from build123d import *

# Parameters (mm, degrees)
SKETCH2_R           = 42.5
BOSS_EXTRUDE2_DEPTH = 75
SKETCH3_R           = 27.5
BOSS_EXTRUDE3_DEPTH = 40
SKETCH4_W           = 10.5
SKETCH4_H           = 8.79879656
CUT_EXTRUDE1_DEPTH  = 50


with BuildPart() as part:
    # Sketch2 → Boss-Extrude2 (new, symmetric)
    with BuildSketch(Plane.XY):
        Circle(SKETCH2_R)
    extrude(amount=BOSS_EXTRUDE2_DEPTH, both=True)

    # Sketch3 → Boss-Extrude3 (add)
    with BuildSketch(Plane.XY.offset(75)):
        Circle(SKETCH3_R)
    boss_extrude3 = extrude(amount=BOSS_EXTRUDE3_DEPTH)

    # Sketch4 → Cut-Extrude1 (cut, symmetric)
    with BuildSketch(Plane(origin=(0, 0, 0), x_dir=(0, 0, -1), z_dir=(1, 0, 0))):
        with Locations((-96.25, 24.39939828)):
            Rectangle(SKETCH4_W, SKETCH4_H)
    cut_extrude1 = extrude(amount=CUT_EXTRUDE1_DEPTH, both=True, mode=Mode.SUBTRACT)

    # Mirror3: Boss-Extrude3, Cut-Extrude1 across plane
    add(boss_extrude3.mirror(Plane.XY))
    add(cut_extrude1.mirror(Plane.XY), mode=Mode.SUBTRACT)


solid = part.part
Source: CAD feature listing. Evaluate the final solid. Frame: model axes, mm. A direction names the side the tool comes from. Round coordinates to 2 decimals unless told otherwise and drop trailing zeros. Order: outer loops, then holes, each group sorted by start corner. A loop starts at its lowest first (then second) coordinate and runs counter-clockwise, first axis right, second up. Notation, with made-up numbers: (61.5, 4.5) - (120.5, 4.5) arc R19 ccw to (120.5, 19.5) - close; hole circle Ø11 at (73, 14). An arc over 180 degrees is marked (long way). Use a Markdown table: item, result. Add a question column.
1. Set-up query: faces 4 (the flat face through (0, 0, -115)), 5 (the flat face through (0, 23, -101.5)), 6 (the cylindrical face through (-5.961, -26.846, 94.72)), 7 (the cylindrical face through (-5.961, -26.846, -94.72)). Return all of +Z, -Z, +X, -X, +Y, -Y with unobstructed straight access to the full face (end or side cutting, diameter ignored); none if empty.
2. First-contact query: pin 1 (3 mm diameter, centred on x = -31.5, y = 4.5, fed in from +Z); pin 2 (6 mm diameter, centred on y = 30.5, z = 6, fed in from +X); pin 3 (1 mm diameter, centred on y = 6.5, z = 87, fed in from -X). Flat tips, straight axial feed; report the tip coordinate or a pass-through.
3. Section query C-C (z = 54.5). Return the cut outline in (x, y), then the cut area to 3 significant figures.
4. Section query A-A (x = 0). Return the cut outline in (y, z).
5. Line query: probe 1 along Z at (x, y) = (-14, 21); probe 2 along Y at (x, z) = (1, 100.5); probe 3 along Z at (x, y) = (-28, -20). Output: solid intervals per line, ascending.
6. Mould query, pull axis Z, two halves, no side actions, for faces 1 (the flat face through (0, 23, -91)), 2 (the flat face through (-1, -28, -75)), 3 (the flat face through (0, 0, 115)). Classes: +Z half, -Z half, draft (parallel to the pull), parting line (faces both ways), or undercut.
7. Section query D-D (x = 21.5). Return the cut outline in (y, z).
8. Section query B-B (y = 0). Return the cut outline in (x, z), then the cut area to 4 significant figures.
Derived:
| question | item | result |
|---|---|---|
| 1 | face 4 | -Z, +X, -X, +Y, -Y |
| 1 | face 5 | +X, -X, +Y |
| 1 | face 6 | +Z |
| 1 | face 7 | -Z |
| 2 | pin 1 | z = 75 |
| 2 | pin 2 | x = 32.4 |
| 2 | pin 3 | x = -26.84 |
| 3 | outline | circle Ø85 at (0, 0) |
| 3 | area | 5,670 mm2 |
| 4 | outline | (-42.5, -75) - (-27.5, -75) - (-27.5, -115) - (27.5, -115) - (27.5, -101.5) - (20, -101.5) - (20, -91) - (27.5, -91) - (27.5, -75) - (42.5, -75) - (42.5, 75) - (27.5, 75) - (27.5, 91) - (20, 91) - (20, 101.5) - (27.5, 101.5) - (27.5, 115) - (-27.5, 115) - (-27.5, 75) - (-42.5, 75) - close |
| 5 | probe 1 | -115 to -101.5, -91 to 91, 101.5 to 115 |
| 5 | probe 2 | -27.48 to 20 |
| 5 | probe 3 | -75 to 75 |
| 6 | face 1 | undercut |
| 6 | face 2 | -Z half |
| 6 | face 3 | +Z half |
| 7 | outline | (-36.66, -75) - (-17.15, -75) - (-17.15, -115) - (17.15, -115) - (17.15, -75) - (36.66, -75) - (36.66, 75) - (17.15, 75) - (17.15, 115) - (-17.15, 115) - (-17.15, 75) - (-36.66, 75) - close |
| 8 | outline | (-42.5, -75) - (-27.5, -75) - (-27.5, -115) - (27.5, -115) - (27.5, -75) - (42.5, -75) - (42.5, 75) - (27.5, 75) - (27.5, 115) - (-27.5, 115) - (-27.5, 75) - (-42.5, 75) - close |
| 8 | area | 17,150 mm2 |
